Solid Edge part; units mm, degrees
sketch "Sketch1" plane through (0, 0, 0) normal (0, 0, 1) x (1, 0, 0)
  circle A0 centre (0, 0) radius 7.1374
extrude "Protrusion1" add sketch "Sketch1" along normal blind 6.35
sketch "Sketch2" plane through (0, 0, 0) normal (0, 0, -1) x (0, 1, 0)
  circle A0 centre (0, 0) radius 4.7625
extrude "Protrusion2" add sketch "Sketch2" along normal blind 25.4
sketch "Sketch3" plane through (0, 0, -25.4) normal (0, 0, -1) x (0, 1, 0)
  circle A0 centre (0, 0) radius 3.9688
extrude "Protrusion3" add sketch "Sketch3" along normal blind 12.7
sketch "Sketch4" plane through (0, 0, 6.35) normal (0, 0, 1) x (0, 1, 0)
  line L0 (-2.3876, 1.3131) -> (0, 2.8792)
  line L1 (-2.3876, -1.5424) -> (-2.3876, 1.3131)
  line L2 (-2.3876, -1.5424) -> (0, -2.8792)
  line L3 (2.3876, -1.5424) -> (0, -2.8792)
  line L4 (2.3876, -1.5424) -> (2.3876, 1.3131)
  line L5 (2.3876, 1.3131) -> (0, 2.8792)
extrude "Cutout1" cut sketch "Sketch4" against normal blind 3.175
chamfer "Chamfer1" distance 0.7874 angle 45 1 edges at (0, -3.9688, -38.1)
properties part number "171469" material "Stainless Steel, 304"
CAD build for the part. Positions are in the model's coordinates, mm. A direction names the side the tool comes from. Coordinates: 2 decimals unless noted, no trailing zeros. Order: outer loops, then holes, each group sorted by start corner. A loop starts at its lowest first (then second) coordinate and runs counter-clockwise, first axis right, second up. Notation, with made-up numbers: (-5, 84) -> (22, 84) arc R17 ccw to (22, 93) -> close; hole circle Ø9 at (20, 42). An arc over 180 degrees is marked (long way). Use one line per item in the form item = value. Start each with the question number.
1) Band-saw the part on B-B on z = -16.5. Give the cut face in (x, y) (1 decimal), then the cut area to 3 significant figures.
2) Band-saw the part on D-D on x = 5.5. Give the cut face in (y, z), then the cut area to 3 significant figures.
3) Drop flat-ended pins along their axis: pin 1 (1 mm diameter, centred on y = 5, z = -27, fed in from -X); pin 2 (1.5 mm diameter, centred on x = 2, y = -5.5, fed in from -Z); pin 3 (4 mm diameter, centred on x = -0.5, y = -0.5, fed in from +Z); pin 4 (6 mm diameter, centred on y = -4.5, z = -10, fed in from +X). Give the stop position or say it passes through.
4) Tool access for faces 5 (the cylindrical face through (1.52, 3.666, -31.273)), 6 (the flat face through (0, -3, 6.35)), 7 (the flat face through (2.2, 1.21, 4.78)): list every direction of +Z, -Z, +X, -X, +Y, -Y with a clear straight run to the whole face (end or side of a thin tool).
5) Drill centre lines: L1, parallel to Z at x = 5, y = 3.5; L2, parallel to Z at x = 1.5, y = 2.25 (3 decimals); L3, parallel to Y at x = -1.25, z = -28. Where is each one in solid material? Low to high. Write a range as [from, to].
6) Pull direction Y, two halves, no side cores. Call faces 1 (the cylindrical face through (-7.13, -0.31, 3.13)), 2 (the flat face through (2, 4, -25.4)), 3 (the flat face through (0, 2.388, 5)), 4 (the flat face through (0, 0, 3.175)): +Y half, -Y half, draft (parallel to the pull), parting line (faces both ways), or undercut.
7) Band-saw the part on C-C on z = -29. Give the cut face in (x, y), then the cut area to 3 significant figures.
Entries:
q1.outline = circle Ø9.5 at (0, 0)
q1.area = 71.3 mm2
q2.outline = (-4.55, 0) -> (4.55, 0) -> (4.55, 6.35) -> (-4.55, 6.35) -> close
q2.area = 57.8 mm2
q3.pin_1 = through
q3.pin_2 = 0
q3.pin_3 = 6.35
q3.pin_4 = 4.52
q4.face_5 = -Z
q4.face_6 = +Z, +X, -X, +Y, -Y
q4.face_7 = +Z
q5.L1 = [0, 6.35]
q5.L2 = [-38.1, 3.175]
q5.L3 = [-3.77, 3.77]
q6.face_1 = parting line
q6.face_2 = draft
q6.face_3 = undercut
q6.face_4 = undercut
q7.outline = circle Ø7.94 at (0, 0)
q7.area = 49.5 mm2
